```python
from build123d import *

# Parameters (mm, degrees)
SKETCH1_W           = 26
SKETCH1_H           = 50
SKETCH1_R           = 1.35
BOSS_EXTRUDE1_DEPTH = 1
BOSS_EXTRUDE2_DEPTH = 5
FILLET1_R           = 1
FILLET2_R           = 5
SKETCH3_R           = 2.625
CUT_EXTRUDE1_DEPTH  = 3


with BuildPart() as part:
    # Sketch1 → Boss-Extrude1 (new body)
    with BuildSketch(Plane.XY):
        Rectangle(SKETCH1_W, SKETCH1_H)
        with Locations((10, -21)):
            Circle(SKETCH1_R, mode=Mode.SUBTRACT)
        with Locations((10, -7)):
            Circle(SKETCH1_R, mode=Mode.SUBTRACT)
        with Locations((10, 7)):
            Circle(SKETCH1_R, mode=Mode.SUBTRACT)
        with Locations((10, 21)):
            Circle(SKETCH1_R, mode=Mode.SUBTRACT)
        with Locations((-10, -7)):
            Circle(SKETCH1_R, mode=Mode.SUBTRACT)
        with Locations((-10, 7)):
            Circle(SKETCH1_R, mode=Mode.SUBTRACT)
        with Locations((-10, 21)):
            Circle(SKETCH1_R, mode=Mode.SUBTRACT)
        with Locations((-10, -21)):
            Circle(SKETCH1_R, mode=Mode.SUBTRACT)
    extrude(amount=BOSS_EXTRUDE1_DEPTH)

    # Sketch2 → Boss-Extrude2 (add)
    with BuildSketch(Plane.XY.offset(1)):
        with BuildLine():
            Line((-2.5, 24.5), (2.5, 24.5))
            ThreePointArc((2.5, 24.5), (6, 21), (2.5, 17.5))
            Line((2.5, 17.5), (-2.5, 17.5))
            ThreePointArc((-2.5, 17.5), (-6, 21), (-2.5, 24.5))
        make_face()
        with BuildLine():
            Line((-2.5, 3.5), (2.5, 3.5))
            ThreePointArc((2.5, 3.5), (6, 7), (2.5, 10.5))
            Line((2.5, 10.5), (-2.5, 10.5))
            ThreePointArc((-2.5, 10.5), (-6, 7), (-2.5, 3.5))
        make_face()
        with BuildLine():
            Line((-2.5, -10.5), (2.5, -10.5))
            ThreePointArc((2.5, -10.5), (6, -7), (2.5, -3.5))
            Line((2.5, -3.5), (-2.5, -3.5))
            ThreePointArc((-2.5, -3.5), (-6, -7), (-2.5, -10.5))
        make_face()
        with BuildLine():
            Line((-2.5, -24.5), (2.5, -24.5))
            ThreePointArc((2.5, -24.5), (6, -21), (2.5, -17.5))
            Line((2.5, -17.5), (-2.5, -17.5))
            ThreePointArc((-2.5, -17.5), (-6, -21), (-2.5, -24.5))
        make_face()
    extrude(amount=BOSS_EXTRUDE2_DEPTH)

    # Fillet1
    fillet1_edges = [part.edges().sort_by_distance(p)[0] for p in [
        (-6, 21, 6),
        (0, 17.5, 6),
        (6, 21, 6),
        (0, 24.5, 6),
        (-6, 7, 6),
        (0, 3.5, 6),
        (6, 7, 6),
        (0, 10.5, 6),
        (-6, -7, 6),
        (0, -10.5, 6),
        (6, -7, 6),
        (0, -3.5, 6),
        (-6, -21, 6),
        (0, -24.5, 6),
        (6, -21, 6),
        (0, -17.5, 6),
    ]]
    fillet(fillet1_edges, radius=FILLET1_R)

    # Fillet2
    fillet2_edges = [part.edges().sort_by_distance(p)[0] for p in [
        (-13, 25, 0.5),
        (13, 25, 0.5),
        (13, -25, 0.5),
        (-13, -25, 0.5),
    ]]
    fillet(fillet2_edges, radius=FILLET2_R)

    # Sketch3 → Cut-Extrude1 (cut)
    with BuildSketch(Plane(origin=(0, 0, 0), x_dir=(-1, 0, 0), z_dir=(0, 0, -1))):
        with Locations((0, 21)):
            Circle(SKETCH3_R)
        with Locations((0, 7)):
            Circle(SKETCH3_R)
        with Locations((0, -7)):
            Circle(SKETCH3_R)
        with Locations((0, -21)):
            Circle(SKETCH3_R)
    extrude(amount=-CUT_EXTRUDE1_DEPTH, mode=Mode.SUBTRACT)


solid = part.part
```
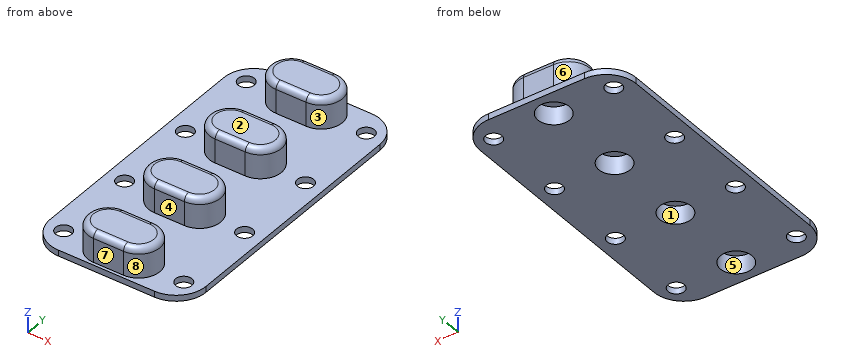
Check sheet for the modelled part. Datum: model origin and axes. Units: mm. Face numbers are marked on the shaded views. A direction names the side the tool comes from. Coordinates: 2 decimals unless noted, no trailing zeros. Loops run counter-clockwise (first coordinate to the right, second up) from the corner with the lowest first, then second, coordinate; pieces in that order, holes last.
1) Sectioned sample at B-B (x = -10). Record the boundary of the cut face in (y, z), and give its area (3 significant figures).
2) Sectioned sample at D-D (y = -1). Record the boundary of the cut face in (x, z), and give its area (3 significant figures).
3) Sectioned sample at A-A (z = 1.9). Record the boundary of the cut face in (x, y) (3 decimals).
4) Material ranges on probe 1 along Y at (x, z) = (-5.25, 3); probe 2 along Z at (x, y) = (-4.75, -12); probe 3 along Y at (x, z) = (-10, 0.45), recorded low to high.
5) Release check for a two-part mould opening along X. For the marked faces 1, 2 and 3 record: released by +X, released by -X, zero draft, split by the parting line, or undercut.
6) Gauge pin test, flat ends, axial feed: pin 1 (2 mm diameter, centred on x = 1, z = 3, fed in from -Y); pin 2 (4 mm diameter, centred on x = 0, y = -7, fed in from -Z); pin 3 (2 mm diameter, centred on x = -9.5, y = 14.5, fed in from +Z). Record the tip position at first contact, or that the pin passes through.
7) Access from +Z, -Z, +X, -X, +Y, -Y to the whole of each face (thin tool, end or side, straight path). Record for the marked faces 4, 5, 6, 7 and 8.
8) Sectioned sample at C-C (y = -7). Record the boundary of the cut face in (x, z) (3 decimals).
Check sheet entries:
1. outline: (-24.58, 0) - (-22.35, 0) - (-22.35, 1) - (-24.58, 1) - close; (-19.65, 0) - (-8.35, 0) - (-8.35, 1) - (-19.65, 1) - close; (-5.65, 0) - (5.65, 0) - (5.65, 1) - (-5.65, 1) - close; (8.35, 0) - (19.65, 0) - (19.65, 1) - (8.35, 1) - close; (22.35, 0) - (24.58, 0) - (24.58, 1) - (22.35, 1) - close
1. area: 38.4 mm2
2. outline: (-13, 0) - (13, 0) - (13, 1) - (-13, 1) - close
2. area: 26.0 mm2
3. outline: (-2.5, -24.5) - (2.5, -24.5) arc R3.5 ccw to (2.5, -17.5) - (-2.5, -17.5) arc R3.5 ccw to start; (-2.5, -10.5) - (2.5, -10.5) arc R3.5 ccw to (2.5, -3.5) - (-2.5, -3.5) arc R3.5 ccw to start; (-2.5, 3.5) - (2.5, 3.5) arc R3.5 ccw to (2.5, 10.5) - (-2.5, 10.5) arc R3.5 ccw to start; (-2.5, 17.5) - (2.5, 17.5) arc R3.5 ccw to (2.5, 24.5) - (-2.5, 24.5) arc R3.5 ccw to start; hole circle Ø5.25 at (0, -21); hole circle Ø5.25 at (0, -7); hole circle Ø5.25 at (0, 7); hole circle Ø5.25 at (0, 21)
4. probe 1: y = -23.17 to -18.83, -9.17 to -4.83, 4.83 to 9.17, 18.83 to 23.17
4. probe 2: z = 0 to 1
4. probe 3: y = -24.58 to -22.35, -19.65 to -8.35, -5.65 to 5.65, 8.35 to 19.65, 22.35 to 24.58
5. face 1: undercut
5. face 2: zero draft
5. face 3: released by +X
6. pin 1: stops at y = -24.5
6. pin 2: stops at z = 3
6. pin 3: stops at z = 1
7. face 4: +Z, +X, -X
7. face 5: -Z
7. face 6: +Z, -X
7. face 7: +Z, +X, -X, -Y
7. face 8: +Z, +X
8. outline: (-13, 0) - (-11.35, 0) - (-11.35, 1) - (-13, 1) - close; (-8.65, 0) - (-2.625, 0) - (-2.625, 3) - (2.625, 3) - (2.625, 0) - (8.65, 0) - (8.65, 1) - (6, 1) - (6, 5) arc R1 ccw to (5, 6) - (-5, 6) arc R1 ccw to (-6, 5) - (-6, 1) - (-8.65, 1) - close; (11.35, 0) - (13, 0) - (13, 1) - (11.35, 1) - close
